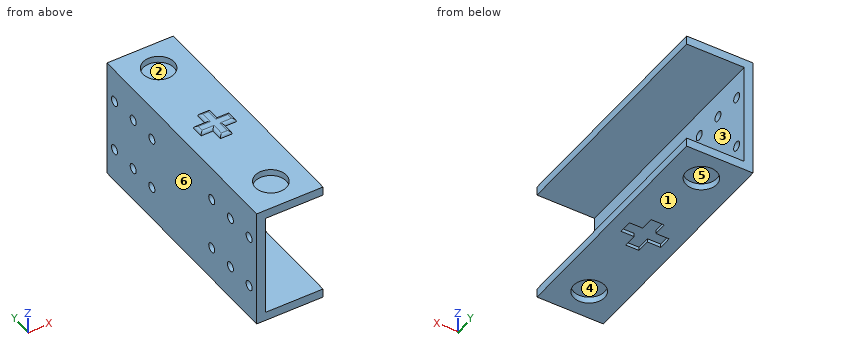
```python
from build123d import *

# Parameters (mm, degrees)
ESQUISSE1_W             = 22.5
ESQUISSE1_H             = 80
BOSS_EXTRU_1_DEPTH      = 3
ESQUISSE2_W             = 3
ESQUISSE2_H             = 80
BOSS_EXTRU_2_DEPTH      = 35
ESQUISSE3_W             = 22.5
ESQUISSE3_H             = 80
BOSS_EXTRU_3_DEPTH      = 3
ESQUISSE4_R             = 5.25
ENL_V_MAT_EXTRU_1_DEPTH = 2.2
ENL_V_START             = -1.8
ENL_V_MAT_EXTRU_2_DEPTH = 1.2
ENL_V_START_2           = -2.2
ESQUISSE6_R             = 5.25
ENL_V_MAT_EXTRU_3_DEPTH = 2.2
BOSS_EXTRU_4_DEPTH      = 1
ESQUISSE8_R             = 1.6
ENL_V_MAT_EXTRU_4_DEPTH = 4
CONG_2_R                = 1


with BuildPart() as part:
    # Esquisse1 → Boss.-Extru.1 (new body)
    with BuildSketch(Plane.XY):
        with Locations((11.25, 40)):
            Rectangle(ESQUISSE1_W, ESQUISSE1_H)
    extrude(amount=BOSS_EXTRU_1_DEPTH)

    # Esquisse2 → Boss.-Extru.2 (add)
    with BuildSketch(Plane.XY.offset(3)):
        with Locations((1.5, 40)):
            Rectangle(ESQUISSE2_W, ESQUISSE2_H)
    extrude(amount=BOSS_EXTRU_2_DEPTH)

    # Esquisse3 → Boss.-Extru.3 (add)
    with BuildSketch(Plane.XY.offset(38)):
        with Locations((11.25, 40)):
            Rectangle(ESQUISSE3_W, ESQUISSE3_H)
    extrude(amount=BOSS_EXTRU_3_DEPTH)

    # Esquisse4 → Enlèv. mat.-Extru.1 (cut)
    with BuildSketch(Plane(origin=(0, 0, 0), x_dir=(-1, 0, 0), z_dir=(0, 0, -1))):
        with Locations((-11.25, 10.15)):
            Circle(ESQUISSE4_R)
        with Locations((-11.25, 70.15)):
            Circle(ESQUISSE4_R)
    extrude(amount=-ENL_V_MAT_EXTRU_1_DEPTH, mode=Mode.SUBTRACT)

    # Esquisse5 → Enlèv. mat.-Extru.2 (cut)
    with BuildSketch(Plane.XY.offset(3).offset(ENL_V_START)):
        Polygon((4.5, 37.75), (9, 37.75), (9, 33.25), (13.5, 33.25), (13.5, 37.75), (18, 37.75), (18, 42.25), (13.5, 42.25), (13.5, 46.75), (9, 46.75), (9, 42.25), (4.5, 42.25), align=None)
    extrude(amount=-ENL_V_MAT_EXTRU_2_DEPTH, mode=Mode.SUBTRACT)

    # Esquisse6 → Enlèv. mat.-Extru.3 (cut)
    with BuildSketch(Plane.XY.offset(41).offset(ENL_V_START_2)):
        with Locations(Location((11.25, 10.15, 0), (0, 0, 180))):
            Circle(ESQUISSE6_R)
        with Locations(Location((11.25, 70.15, 0), (0, 0, 180))):
            Circle(ESQUISSE6_R)
    extrude(amount=ENL_V_MAT_EXTRU_3_DEPTH, mode=Mode.SUBTRACT)

    # Esquisse7 → Boss.-Extru.4 (add)
    with BuildSketch(Plane.XY.offset(41)):
        Polygon((5.25, 42), (9.25, 42), (9.25, 46), (13.25, 46), (13.25, 42), (17.25, 42), (17.25, 38), (13.25, 38), (13.25, 34), (9.25, 34), (9.25, 38), (5.25, 38), align=None)
    extrude(amount=BOSS_EXTRU_4_DEPTH)

    # Esquisse8 → Enlèv. mat.-Extru.4 (cut)
    with BuildSketch(Plane.ZY):
        with Locations((29.5, 76)):
            Circle(ESQUISSE8_R)
        with Locations((29.5, 66)):
            Circle(ESQUISSE8_R)
        with Locations((29.5, 56)):
            Circle(ESQUISSE8_R)
        with Locations((11.5, 76)):
            Circle(ESQUISSE8_R)
        with Locations((11.5, 66)):
            Circle(ESQUISSE8_R)
        with Locations((11.5, 56)):
            Circle(ESQUISSE8_R)
        with Locations((11.5, 4)):
            Circle(ESQUISSE8_R)
        with Locations((11.5, 14)):
            Circle(ESQUISSE8_R)
        with Locations((11.5, 24)):
            Circle(ESQUISSE8_R)
        with Locations((29.5, 24)):
            Circle(ESQUISSE8_R)
        with Locations((29.5, 14)):
            Circle(ESQUISSE8_R)
        with Locations((29.5, 4)):
            Circle(ESQUISSE8_R)
    extrude(amount=-ENL_V_MAT_EXTRU_4_DEPTH, mode=Mode.SUBTRACT)

    # Congé2
    cong_2_edges = [part.edges().sort_by_distance(p)[0] for p in [
        (11.25, 46, 42),
        (9.25, 44, 42),
        (13.25, 44, 42),
        (15.25, 42, 42),
        (17.25, 40, 42),
        (15.25, 38, 42),
        (13.25, 36, 42),
        (9.25, 36, 42),
        (7.25, 38, 42),
        (7.25, 42, 42),
        (5.25, 40, 42),
        (11.25, 34, 42),
    ]]
    fillet(cong_2_edges, radius=CONG_2_R - 0.0001)  # a hair under: the kernel refuses the full size


solid = part.part
```
Check sheet for the modelled part. Datum: model origin and axes. Units: mm. Face numbers are marked on the shaded views. A direction names the side the tool comes from. Give positions to 0.01 mm unless a question says otherwise; leave off trailing zeros. Loops run counter-clockwise (first coordinate to the right, second up) from the corner with the lowest first, then second, coordinate; pieces in that order, holes last. Notation, with made-up numbers: (62, 28.25) - (120, 28.25) arc R17 cw to (120, 53.25) - close; hole circle Ø1 at (-11.75, 57). An arc over 180 degrees is marked (long way). One line per question, with ' | ' between items. Start each with the question number.
1. Cross-section at A-A, the plane y = 4. Enter the section's corners in (x, z), plus the area to 3 significant figures.
2. Material ranges on line 1 along Y through (x, z) = (11.25, 40.1); line 2 along Z through (x, y) = (1, 66); line 3 along Z through (x, y) = (17, 33), recorded low to high. Write a range as [from, to].
3. Set-up check for the marked faces 1, 2, 3 and 4: record each of +Z, -Z, +X, -X, +Y, -Y from which the full face is reachable in a straight line by a thin tool's end or side.
4. Gauge pin test, flat ends, axial feed: pin 1 Ø5 at (x, y) = (15.5, 64) entering from +Z; pin 2 Ø6 at (y, z) = (37.5, 12.5) entering from +X. Record the tip position at first contact, or that the pin passes through.
5. Cross-section at B-B, the plane z = 29.5. Enter the section's corners in (x, y).
6. Cross-section at C-C, the plane y = 27.5. Enter the section's corners in (x, z), plus the area to 3 significant figures.
7. Draft check along Y on the marked faces 5 and 6. Enter one of: released by +Y, released by -Y, zero draft, split by the parting line, or undercut.
Check result:
1) outline: (0, 0) - (22.5, 0) - (22.5, 3) - (3, 3) - (3, 9.9) - (0, 9.9) - close; (0, 13.1) - (3, 13.1) - (3, 27.9) - (0, 27.9) - close; (0, 31.1) - (3, 31.1) - (3, 38) - (22.5, 38) - (22.5, 41) - (0, 41) - close | area: 221 mm2
2) line 1: y = [0, 4.9], [15.4, 64.9], [75.4, 80] | line 2: z = [0, 9.9], [13.1, 27.9], [31.1, 41] | line 3: z = [0, 3], [38, 41]
3) face 1: -Z, +X, -X, +Y, -Y | face 2: +Z | face 3: +X, +Y, -Y | face 4: -Z
4) pin 1: stops at z = 41 | pin 2: stops at x = 3
5) outline: (0, 0) - (3, 0) - (3, 2.4) - (0, 2.4) - close; (0, 5.6) - (3, 5.6) - (3, 12.4) - (0, 12.4) - close; (0, 15.6) - (3, 15.6) - (3, 22.4) - (0, 22.4) - close; (0, 25.6) - (3, 25.6) - (3, 54.4) - (0, 54.4) - close; (0, 57.6) - (3, 57.6) - (3, 64.4) - (0, 64.4) - close; (0, 67.6) - (3, 67.6) - (3, 74.4) - (0, 74.4) - close; (0, 77.6) - (3, 77.6) - (3, 80) - (0, 80) - close
6) outline: (0, 0) - (22.5, 0) - (22.5, 3) - (3, 3) - (3, 38) - (22.5, 38) - (22.5, 41) - (0, 41) - close | area: 240 mm2
7) face 5: undercut | face 6: zero draft
